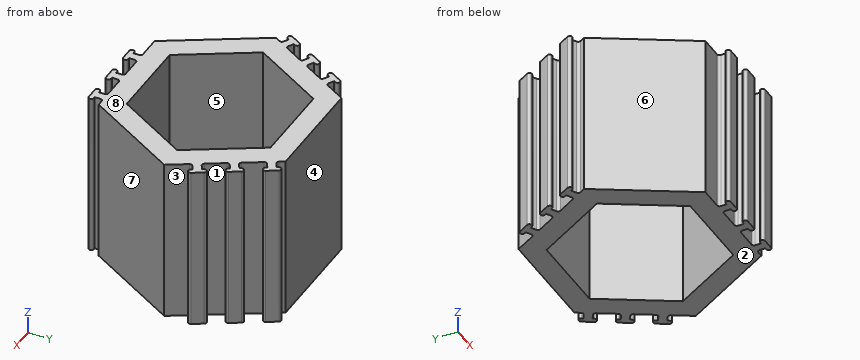
```python
from build123d import *

# Parameters (mm, degrees)
F1_DEPTH = 100


with BuildPart() as f1:
    # F0 (on Top) → F1 (new body)
    with BuildSketch(Plane.XY):
        with BuildLine():
            Line((-63.261107, 3.031089), (-65.011107, 0))
            Line((-65.011107, 0), (-32.505553, -56.30127))
            Line((-32.505553, -56.30127), (-18.994447, -56.30127))
            Line((-18.994447, -56.30127), (-10.994447, -56.30127))
            Line((-10.994447, -56.30127), (1.005553, -56.30127))
            Line((1.005553, -56.30127), (9.005553, -56.30127))
            Line((9.005553, -56.30127), (21.005553, -56.30127))
            Line((21.005553, -56.30127), (29.005553, -56.30127))
            Line((29.005553, -56.30127), (32.505553, -56.30127))
            Line((32.505553, -56.30127), (65.011107, 0))
            Line((65.011107, 0), (58.255553, 11.700962))
            Line((58.255553, 11.700962), (54.255553, 18.629165))
            Line((54.255553, 18.629165), (48.255553, 29.02147))
            Line((48.255553, 29.02147), (44.255553, 35.949673))
            Line((44.255553, 35.949673), (38.255553, 46.341978))
            ThreePointArc((38.255553, 46.341978), (38.105703, 47.480207), (38.804592, 48.391016))
            Line((38.804592, 48.391016), (41.835681, 50.141016))
            Line((41.835681, 50.141016), (42.335681, 49.274991))
            ThreePointArc((42.335681, 49.274991), (43.24649, 48.576102), (44.384719, 48.725953))
            ThreePointArc((44.384719, 48.725953), (45.083607, 49.636762), (44.933757, 50.774991))
            Line((44.933757, 50.774991), (41.433757, 56.837169))
            ThreePointArc((41.433757, 56.837169), (40.522947, 57.536057), (39.384719, 57.386207))
            ThreePointArc((39.384719, 57.386207), (38.68583, 56.475397), (38.835681, 55.337169))
            Line((38.835681, 55.337169), (39.335681, 54.471143))
            Line((39.335681, 54.471143), (36.304592, 52.721143))
            ThreePointArc((36.304592, 52.721143), (35.166363, 52.571293), (34.255553, 53.270181))
            Line((34.255553, 53.270181), (32.505553, 56.30127))
            Line((32.505553, 56.30127), (-32.505553, 56.30127))
            Line((-32.505553, 56.30127), (-39.261107, 44.600308))
            Line((-39.261107, 44.600308), (-43.261107, 37.672105))
            Line((-43.261107, 37.672105), (-49.261107, 27.2798))
            Line((-49.261107, 27.2798), (-53.261107, 20.351597))
            Line((-53.261107, 20.351597), (-59.261107, 9.959292))
            Line((-59.261107, 9.959292), (-63.261107, 3.031089))
        make_face()
        Polygon((-50, 0), (-25, 43.30127), (25, 43.30127), (50, 0), (25, -43.30127), (-25, -43.30127), align=None, mode=Mode.SUBTRACT)
        with BuildLine():
            ThreePointArc((-63.810145, 5.080127), (-63.111256, 4.169317), (-63.261107, 3.031089))
            Line((-63.261107, 3.031089), (-59.261107, 9.959292))
            ThreePointArc((-59.261107, 9.959292), (-60.171917, 9.260403), (-61.310145, 9.410254))
            Line((-61.310145, 9.410254), (-64.341234, 11.160254))
            Line((-64.341234, 11.160254), (-63.841234, 12.026279))
            ThreePointArc((-63.841234, 12.026279), (-63.691383, 13.164508), (-64.390272, 14.075318))
            ThreePointArc((-64.390272, 14.075318), (-65.528501, 14.225168), (-66.43931, 13.526279))
            Line((-66.43931, 13.526279), (-69.93931, 7.464102))
            ThreePointArc((-69.93931, 7.464102), (-70.089161, 6.325873), (-69.390272, 5.415064))
            ThreePointArc((-69.390272, 5.415064), (-68.252044, 5.265213), (-67.341234, 5.964102))
            Line((-67.341234, 5.964102), (-66.841234, 6.830127))
            Line((-66.841234, 6.830127), (-63.810145, 5.080127))
        make_face()
        with BuildLine():
            Line((-10.994447, -56.30127), (-18.994447, -56.30127))
            ThreePointArc((-18.994447, -56.30127), (-17.933786, -56.74061), (-17.494447, -57.80127))
            Line((-17.494447, -57.80127), (-17.494447, -61.30127))
            Line((-17.494447, -61.30127), (-18.494447, -61.30127))
            ThreePointArc((-18.494447, -61.30127), (-19.555107, -61.74061), (-19.994447, -62.80127))
            ThreePointArc((-19.994447, -62.80127), (-19.555107, -63.86193), (-18.494447, -64.30127))
            Line((-18.494447, -64.30127), (-11.494447, -64.30127))
            ThreePointArc((-11.494447, -64.30127), (-10.433786, -63.86193), (-9.994447, -62.80127))
            ThreePointArc((-9.994447, -62.80127), (-10.433786, -61.74061), (-11.494447, -61.30127))
            Line((-11.494447, -61.30127), (-12.494447, -61.30127))
            Line((-12.494447, -61.30127), (-12.494447, -57.80127))
            ThreePointArc((-12.494447, -57.80127), (-12.055107, -56.74061), (-10.994447, -56.30127))
        make_face()
        with BuildLine():
            ThreePointArc((-53.810145, 22.400635), (-53.111256, 21.489826), (-53.261107, 20.351597))
            Line((-53.261107, 20.351597), (-49.261107, 27.2798))
            ThreePointArc((-49.261107, 27.2798), (-50.171917, 26.580911), (-51.310145, 26.730762))
            Line((-51.310145, 26.730762), (-54.341234, 28.480762))
            Line((-54.341234, 28.480762), (-53.841234, 29.346788))
            ThreePointArc((-53.841234, 29.346788), (-53.691383, 30.485016), (-54.390272, 31.395826))
            ThreePointArc((-54.390272, 31.395826), (-55.528501, 31.545676), (-56.43931, 30.846788))
            Line((-56.43931, 30.846788), (-59.93931, 24.78461))
            ThreePointArc((-59.93931, 24.78461), (-60.089161, 23.646381), (-59.390272, 22.735572))
            ThreePointArc((-59.390272, 22.735572), (-58.252044, 22.585721), (-57.341234, 23.28461))
            Line((-57.341234, 23.28461), (-56.841234, 24.150635))
            Line((-56.841234, 24.150635), (-53.810145, 22.400635))
        make_face()
        with BuildLine():
            Line((9.005553, -56.30127), (1.005553, -56.30127))
            ThreePointArc((1.005553, -56.30127), (2.066214, -56.74061), (2.505553, -57.80127))
            Line((2.505553, -57.80127), (2.505553, -61.30127))
            Line((2.505553, -61.30127), (1.505553, -61.30127))
            ThreePointArc((1.505553, -61.30127), (0.444893, -61.74061), (0.005553, -62.80127))
            ThreePointArc((0.005553, -62.80127), (0.444893, -63.86193), (1.505553, -64.30127))
            Line((1.505553, -64.30127), (8.505553, -64.30127))
            ThreePointArc((8.505553, -64.30127), (9.566214, -63.86193), (10.005553, -62.80127))
            ThreePointArc((10.005553, -62.80127), (9.566214, -61.74061), (8.505553, -61.30127))
            Line((8.505553, -61.30127), (7.505553, -61.30127))
            Line((7.505553, -61.30127), (7.505553, -57.80127))
            ThreePointArc((7.505553, -57.80127), (7.944893, -56.74061), (9.005553, -56.30127))
        make_face()
        with BuildLine():
            ThreePointArc((-43.810145, 39.721143), (-43.111256, 38.810334), (-43.261107, 37.672105))
            Line((-43.261107, 37.672105), (-39.261107, 44.600308))
            ThreePointArc((-39.261107, 44.600308), (-40.171917, 43.90142), (-41.310145, 44.05127))
            Line((-41.310145, 44.05127), (-44.341234, 45.80127))
            Line((-44.341234, 45.80127), (-43.841234, 46.667296))
            ThreePointArc((-43.841234, 46.667296), (-43.691383, 47.805524), (-44.390272, 48.716334))
            ThreePointArc((-44.390272, 48.716334), (-45.528501, 48.866184), (-46.43931, 48.167296))
            Line((-46.43931, 48.167296), (-49.93931, 42.105118))
            ThreePointArc((-49.93931, 42.105118), (-50.089161, 40.966889), (-49.390272, 40.05608))
            ThreePointArc((-49.390272, 40.05608), (-48.252044, 39.906229), (-47.341234, 40.605118))
            Line((-47.341234, 40.605118), (-46.841234, 41.471143))
            Line((-46.841234, 41.471143), (-43.810145, 39.721143))
        make_face()
        with BuildLine():
            Line((29.005553, -56.30127), (21.005553, -56.30127))
            ThreePointArc((21.005553, -56.30127), (22.066214, -56.74061), (22.505553, -57.80127))
            Line((22.505553, -57.80127), (22.505553, -61.30127))
            Line((22.505553, -61.30127), (21.505553, -61.30127))
            ThreePointArc((21.505553, -61.30127), (20.444893, -61.74061), (20.005553, -62.80127))
            ThreePointArc((20.005553, -62.80127), (20.444893, -63.86193), (21.505553, -64.30127))
            Line((21.505553, -64.30127), (28.505553, -64.30127))
            ThreePointArc((28.505553, -64.30127), (29.566214, -63.86193), (30.005553, -62.80127))
            ThreePointArc((30.005553, -62.80127), (29.566214, -61.74061), (28.505553, -61.30127))
            Line((28.505553, -61.30127), (27.505553, -61.30127))
            Line((27.505553, -61.30127), (27.505553, -57.80127))
            ThreePointArc((27.505553, -57.80127), (27.944893, -56.74061), (29.005553, -56.30127))
        make_face()
        with BuildLine():
            Line((54.255553, 18.629165), (58.255553, 11.700962))
            ThreePointArc((58.255553, 11.700962), (58.105703, 12.83919), (58.804592, 13.75))
            Line((58.804592, 13.75), (61.835681, 15.5))
            Line((61.835681, 15.5), (62.335681, 14.633975))
            ThreePointArc((62.335681, 14.633975), (63.24649, 13.935086), (64.384719, 14.084936))
            ThreePointArc((64.384719, 14.084936), (65.083607, 14.995746), (64.933757, 16.133975))
            Line((64.933757, 16.133975), (61.433757, 22.196152))
            ThreePointArc((61.433757, 22.196152), (60.522947, 22.895041), (59.384719, 22.745191))
            ThreePointArc((59.384719, 22.745191), (58.68583, 21.834381), (58.835681, 20.696152))
            Line((58.835681, 20.696152), (59.335681, 19.830127))
            Line((59.335681, 19.830127), (56.304592, 18.080127))
            ThreePointArc((56.304592, 18.080127), (55.166363, 17.930276), (54.255553, 18.629165))
        make_face()
        with BuildLine():
            Line((44.255553, 35.949673), (48.255553, 29.02147))
            ThreePointArc((48.255553, 29.02147), (48.105703, 30.159699), (48.804592, 31.070508))
            Line((48.804592, 31.070508), (51.835681, 32.820508))
            Line((51.835681, 32.820508), (52.335681, 31.954483))
            ThreePointArc((52.335681, 31.954483), (53.24649, 31.255594), (54.384719, 31.405445))
            ThreePointArc((54.384719, 31.405445), (55.083607, 32.316254), (54.933757, 33.454483))
            Line((54.933757, 33.454483), (51.433757, 39.51666))
            ThreePointArc((51.433757, 39.51666), (50.522947, 40.215549), (49.384719, 40.065699))
            ThreePointArc((49.384719, 40.065699), (48.68583, 39.154889), (48.835681, 38.01666))
            Line((48.835681, 38.01666), (49.335681, 37.150635))
            Line((49.335681, 37.150635), (46.304592, 35.400635))
            ThreePointArc((46.304592, 35.400635), (45.166363, 35.250784), (44.255553, 35.949673))
        make_face()
    extrude(amount=F1_DEPTH)


solid = f1.part
```
Build history of the part. All positions in model axes, mm. Face numbers are marked on the shaded views. A direction names the side the tool comes from. Round coordinates to 2 decimals unless told otherwise and drop trailing zeros. Write each loop counter-clockwise with the first axis right and the second up, starting at its lowest first coordinate (ties: lowest second). Pieces come first, ordered by that corner, then holes. Notation, with made-up numbers: (86.5, 15.5) - (133.5, 15.5) arc R17 ccw to (133.5, 38.5) - close; hole circle Ø1 at (27.25, 54.5). An arc over 180 degrees is marked (long way). Write each question's results on one line, items separated by ' | '. Start each with the question number.
Item 1: Saw through at C-C (y = -45.5). Write the cut outline in (x, z), and give its area (3 significant figures).
Item 2: Wall check: L1, parallel to X at y = -58, z = 7; L2, parallel to X at y = 37, z = 84.5; L3, parallel to Y at x = -3, z = 93.5. Give the ranges that are in metal, low to high. Write a range as [from, to].
Item 3: Drop flat-ended pins along their axis: P1, Ø4, axis at y = 21, z = 40, coming from the -X side; P2, Ø1.5, axis at x = -30, z = 30.5, coming from the -Y side; P3, Ø8, axis at y = -16.5, z = 55, coming from the +X side. Give the stop position or say it passes through.
Item 4: Saw through at A-A (y = -22.5). Write the cut outline in (x, z).
Item 5: Saw through at B-B (x = -28.5). Write the cut outline in (y, z).
Item 6: Mould opens along X. For the marked faces 5, 6, 7 and 8 say: pulls with the +X half, pulls with the -X half, needs draft (parallel to the pull), parting line crosses it, or undercut.
Item 7: Which spindle directions (+Z, -Z, +X, -X, +Y, -Y) get a long thin tool onto all of the face, cutting with end or side? Do the marked faces 1, 2, 3 and 4. Say none if no direction does.
Results are:
1) outline: (-38.74, 0) - (38.74, 0) - (38.74, 100) - (-38.74, 100) - close | area: 7,750 mm²
2) L1: x = [-17.49, -12.49], [2.51, 7.51], [22.51, 27.51] | L2: x = [-43.65, -28.64], [28.64, 43.65], [49.07, 52.89] | L3: y = [-56.3, -43.3], [43.3, 56.3]
3) P1: stops at x = -59.73 | P2: stops at y = -56.3 | P3: stops at x = 57.79
4) outline: (-52.02, 0) - (-37.01, 0) - (-37.01, 100) - (-52.02, 100) - close; (37.01, 0) - (52.02, 0) - (52.02, 100) - (37.01, 100) - close
5) outline: (-56.3, 0) - (-37.24, 0) - (-37.24, 100) - (-56.3, 100) - close; (37.24, 0) - (56.3, 0) - (56.3, 100) - (37.24, 100) - close
6) face 5: undercut | face 6: pulls with the -X half | face 7: pulls with the +X half | face 8: needs draft
7) face 1: +Z, -Z | face 2: -Z, +X, -X, +Y, -Y | face 3: +Z, -Z, +X | face 4: +Z, -Z, -X, +Y
